Can you work these out from the drawing? Everything is in mm from the part's minimum corner. Give positions to 0.01 mm unless a question says otherwise; leave off trailing zeros. Loops run counter-clockwise (first coordinate to the right, second up) from the corner with the lowest first, then second, coordinate; pieces in that order, holes last. Notation, with made-up numbers: (61, 89.5) - (77, 89.5) arc R23 ccw to (77, 114.5) - close; hole circle Ø3 at (-6, 87). An arc over 180 degrees is marked (long way). Answer in a Markdown table with one row per item.
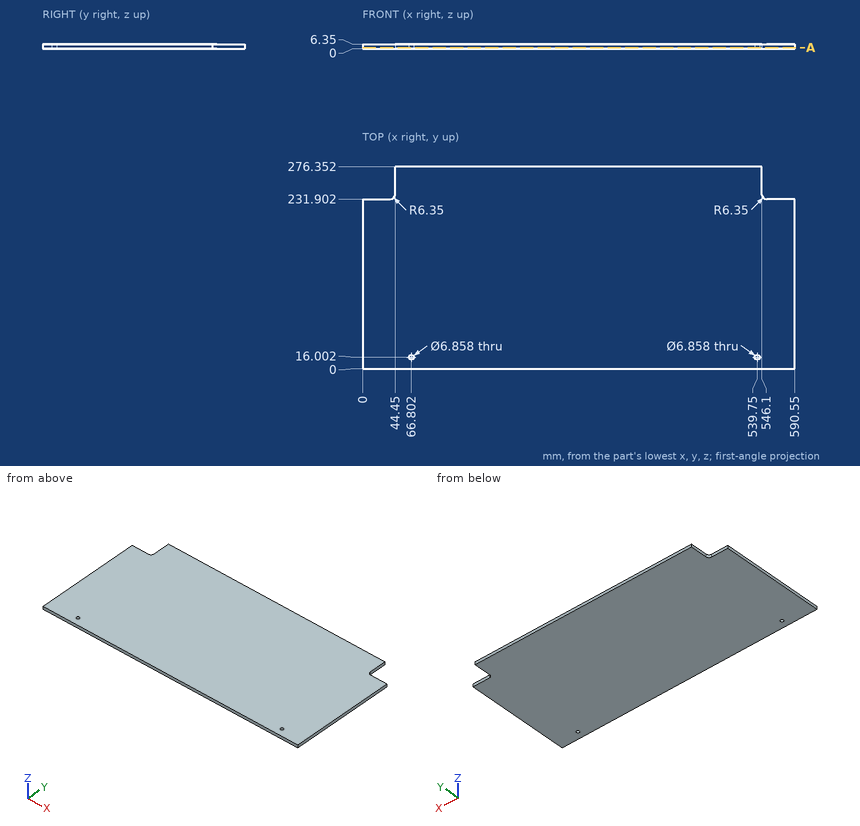
Q1. If I drill on line 1 (Y direction, x = 557, z = 3.75); line 2 (X direction, y = 13, z = 1.75); line 3 (Y direction, x = 539.75, z = 2), over which ranges is the centre line in solid material (lowest first)? Write a range as [from, to].
Checked values:
| item | result |
|---|---|
| line 1 | y = [0, 231.9] |
| line 2 | x = [0, 65.14], [68.46, 538.09], [541.41, 590.55] |
| line 3 | y = [0, 12.57], [19.43, 276.35] |
Q2. Imagine slicing it at A-A, the plane z = 1.5. Write out the boundary of the cut face in (x, y).
Checked values:
| item | result |
|---|---|
| outline | (0, 0) - (590.55, 0) - (590.55, 231.9) - (552.45, 231.9) arc R6.35 cw to (546.1, 238.25) - (546.1, 276.35) - (44.45, 276.35) - (44.45, 238.25) arc R6.35 cw to (38.1, 231.9) - (0, 231.9) - close; hole circle Ø6.86 at (66.8, 16); hole circle Ø6.86 at (539.75, 16) |
Q3. For pin 1 (5.5 mm diameter, centred on x = 66.802, y = 16.002, fed in from -Z); pin 2 (1.9 mm diameter, centred on x = 567, z = 2.5, fed in from +Y); pin 3 (1.9 mm diameter, centred on y = 248.5, z = 4.5, fed in from +X), each with a flat end and sliding along its axis, tell me the tip position at first contact or that it passes through.
Checked values:
| item | result |
|---|---|
| pin 1 | passes through |
| pin 2 | stops at y = 231.9 |
| pin 3 | stops at x = 546.1 |
